CAD build for the part. Positions are in the model's coordinates, mm. Coordinates: 2 decimals unless noted, no trailing zeros. Loops run counter-clockwise (first coordinate to the right, second up) from the corner with the lowest first, then second, coordinate; pieces in that order, holes last. Notation, with made-up numbers: (50.5, 73) -> (95.5, 73) arc R20 ccw to (95.5, 104) -> close; hole circle Ø8 at (-38, -27). An arc over 180 degrees is marked (long way). Write each question's results on one line, items separated by ' | '.
```python
from build123d import *

# Parameters (mm, degrees)
BOSS_EXTRUDE1_DEPTH                             = 6
M3_CLEARANCE_HOLE1_D                            = 3.6
M3_CLEARANCE_HOLE1_DEPTH                        = 6
M3_CLEARANCE_HOLE1_TIP                          = 1.081549114
FILLET1_R                                       = 15
SKETCH4_W                                       = 65
SKETCH4_H                                       = 9
SKETCH4_W_2                                     = 32.5
CUT_EXTRUDE1_DEPTH                              = 2
M4_CLEARANCE_HOLE1_D                            = 4.8
M4_CLEARANCE_HOLE1_DEPTH                        = 6
M4_CLEARANCE_HOLE1_TIP                          = 1.442065486
CHAMFER1_SIZE                                   = 2.4
SKETCH7_W                                       = 65
SKETCH7_H                                       = 78
CUT_EXTRUDE3_DEPTH                              = 132.713704678
FILLET2_R                                       = 15
CSK_FOR_M3_FLAT_HEAD_MACHINE_SCREW1_D           = 3.6
CSK_FOR_M3_FLAT_HEAD_MACHINE_SCREW1_DEPTH       = 20
CSK_FOR_M3_FLAT_HEAD_MACHINE_SCREW1_CSINK_D     = 6.3
CSK_FOR_M3_FLAT_HEAD_MACHINE_SCREW1_CSINK_ANGLE = 90
CSK_FOR_M3_FLAT_HEAD_MACHINE_SCREW1_TIP         = 1.081549114


with BuildPart() as part:
    # Sketch1 → Boss-Extrude1 (new body)
    with BuildSketch(Plane.XY):
        with BuildLine():
            Line((-32.5, 95), (-32.5, -95))
            ThreePointArc((-32.5, -95), (0, -62.5), (32.5, -95))
            Line((32.5, -95), (32.5, 95))
            Line((32.5, 95), (-32.5, 95))
        make_face()
        with BuildLine():
            ThreePointArc((32.5, -95), (0, -62.5), (-32.5, -95))
            Line((-32.5, -95), (-15.5, -95))
            Line((-15.5, -95), (-15.5, -79.5))
            Line((-15.5, -79.5), (15.5, -79.5))
            Line((15.5, -79.5), (15.5, -95))
            Line((15.5, -95), (32.5, -95))
        make_face()
        with BuildLine():
            Line((-15.5, -95), (-32.5, -95))
            ThreePointArc((-32.5, -95), (0, -127.5), (32.5, -95))
            Line((32.5, -95), (15.5, -95))
            Line((15.5, -95), (15.5, -110.5))
            Line((15.5, -110.5), (-15.5, -110.5))
            Line((-15.5, -110.5), (-15.5, -95))
        make_face()
        with BuildLine():
            Line((-14, -95), (-15.5, -95))
            Line((-15.5, -95), (-15.5, -110.5))
            Line((-15.5, -110.5), (15.5, -110.5))
            Line((15.5, -110.5), (15.5, -95))
            Line((15.5, -95), (14, -95))
            ThreePointArc((14, -95), (0, -109), (-14, -95))
        make_face()
        with BuildLine():
            Line((-15.5, -79.5), (-15.5, -95))
            Line((-15.5, -95), (-14, -95))
            ThreePointArc((-14, -95), (0, -81), (14, -95))
            Line((14, -95), (15.5, -95))
            Line((15.5, -95), (15.5, -79.5))
            Line((15.5, -79.5), (-15.5, -79.5))
        make_face()
    extrude(amount=BOSS_EXTRUDE1_DEPTH)

    # M3 Clearance Hole1
    with Locations(Plane(origin=(0, 0, 0), x_dir=(-1, 0, 0), z_dir=(0, 0, -1))):
        with Locations((-15.5, -110.5), (15.5, -110.5), (15.5, -79.5), (-15.5, -79.5)):
            Hole(M3_CLEARANCE_HOLE1_D / 2, depth=M3_CLEARANCE_HOLE1_DEPTH)
            with Locations((0, 0, -(M3_CLEARANCE_HOLE1_DEPTH + M3_CLEARANCE_HOLE1_TIP / 2))):  # 118° drill point
                Cone(0, M3_CLEARANCE_HOLE1_D / 2, M3_CLEARANCE_HOLE1_TIP, mode=Mode.SUBTRACT)

    # Fillet1
    fillet1_edges = [part.edges().sort_by_distance(p)[0] for p in [
        (-32.5, 95, 3),
        (32.5, 95, 3),
    ]]
    fillet(fillet1_edges, radius=FILLET1_R)

    # Sketch4 → Cut-Extrude1 (cut)
    with BuildSketch(Plane.XY.offset(6)):
        with Locations((0, 75.5)):
            Rectangle(SKETCH4_W, SKETCH4_H)
        with Locations((-16.25, 7.5)):
            Rectangle(SKETCH4_W_2, SKETCH4_H)
        with Locations((16.25, 7.5)):
            Rectangle(SKETCH4_W_2, SKETCH4_H)
        with Locations((0, -60.5)):
            Rectangle(SKETCH4_W, SKETCH4_H)
    extrude(amount=-CUT_EXTRUDE1_DEPTH, mode=Mode.SUBTRACT)

    # M4 Clearance Hole1
    with Locations(Plane.XY.offset(4)):
        with Locations((-24.5, -60.5), (-24.5, 75.5), (24.5, 75.5), (0, 75.5), (-24.5, 7.5), (0, 7.5), (24.5, 7.5), (24.5, -60.5), (0, -60.5)):
            Hole(M4_CLEARANCE_HOLE1_D / 2, depth=M4_CLEARANCE_HOLE1_DEPTH)
            with Locations((0, 0, -(M4_CLEARANCE_HOLE1_DEPTH + M4_CLEARANCE_HOLE1_TIP / 2))):  # 118° drill point
                Cone(0, M4_CLEARANCE_HOLE1_D / 2, M4_CLEARANCE_HOLE1_TIP, mode=Mode.SUBTRACT)

    # Chamfer1
    chamfer1_edges = [part.edges().sort_by_distance(p)[0] for p in [
        (-22.1, -60.5, 0),
        (2.4, -60.5, 0),
        (26.9, -60.5, 0),
        (26.9, 7.5, 0),
        (2.4, 7.5, 0),
        (-22.1, 7.5, 0),
        (2.4, 75.5, 0),
        (26.9, 75.5, 0),
        (-22.1, 75.5, 0),
        (13.7, -79.5, 0),
        (-17.3, -79.5, 0),
        (-17.3, -110.5, 0),
        (13.7, -110.5, 0),
    ]]
    chamfer(chamfer1_edges, length=CHAMFER1_SIZE)

    # Sketch7 → Cut-Extrude3 (cut, through all)
    with BuildSketch(Plane.XY.offset(6)):
        with Locations((0, 66)):
            Rectangle(SKETCH7_W, SKETCH7_H)
    extrude(amount=-CUT_EXTRUDE3_DEPTH, mode=Mode.SUBTRACT)

    # Fillet2
    fillet2_edges = [part.edges().sort_by_distance(p)[0] for p in [
        (32.5, 27, 3),
        (-32.5, 27, 3),
    ]]
    fillet(fillet2_edges, radius=FILLET2_R - 0.0001)  # a hair under: the kernel refuses the full size

    # CSK for M3 Flat Head Machine Screw1
    with Locations(Plane(origin=(0, 0, 0), x_dir=(1, 0, 0), z_dir=(0, 0, -1))):
        with Locations((0, 122.3)):
            CounterSinkHole(CSK_FOR_M3_FLAT_HEAD_MACHINE_SCREW1_D / 2, CSK_FOR_M3_FLAT_HEAD_MACHINE_SCREW1_CSINK_D / 2, depth=CSK_FOR_M3_FLAT_HEAD_MACHINE_SCREW1_DEPTH, counter_sink_angle=CSK_FOR_M3_FLAT_HEAD_MACHINE_SCREW1_CSINK_ANGLE)
            with Locations((0, 0, -(CSK_FOR_M3_FLAT_HEAD_MACHINE_SCREW1_DEPTH + CSK_FOR_M3_FLAT_HEAD_MACHINE_SCREW1_TIP / 2))):  # 118° drill point
                Cone(0, CSK_FOR_M3_FLAT_HEAD_MACHINE_SCREW1_D / 2, CSK_FOR_M3_FLAT_HEAD_MACHINE_SCREW1_TIP, mode=Mode.SUBTRACT)


solid = part.part
```
Q1. Drop flat-ended pins along their axis: pin 1 (2.5 mm diameter, centred on x = -3, y = 8, fed in from +Z); pin 2 (0.6 mm diameter, centred on x = -7, z = 4.5, fed in from -Y); pin 3 (22.5 mm diameter, centred on x = 0, y = -95, fed in from +Z); pin 4 (7.5 mm diameter, centred on x = 24.5, y = -60.5, fed in from -Z). Give the stop position or say it passes through.
Results are:
pin 1: z = 4 | pin 2: y = -126.8 | pin 3: through | pin 4: z = 1.05
Q2. Cut at D-D on x = -24. Give the number of separate pieces and of enclosed holes in the cut face, and give its area (3 significant figures).
Results are:
separate pieces: 3 | enclosed holes: 0 | area: 769 mm^2
Q3. Pull direction X, two halves, no side cores. Call faces 1 (the flat face through (-32.5, -41, 3)), 2 (the conical face through (-2.4, 8.26, 2.28)), 3 (the flat face through (0, 27, 3)): +X half, -X half, draft (parallel to the pull), parting line (faces both ways), or undercut.
Results are:
face 1: -X half | face 2: undercut | face 3: draft
Q4. Cut at A-A on y = -60.5. Write the cut outline in (x, z), and give its area (3 significant figures).
Results are:
outline: (-32.5, 0) -> (-29.3, 0) -> (-26.9, 2.4) -> (-26.9, 4) -> (-32.5, 4) -> close; (-22.1, 2.4) -> (-19.7, 0) -> (-4.8, 0) -> (-2.4, 2.4) -> (-2.4, 4) -> (-22.1, 4) -> close; (2.4, 2.4) -> (4.8, 0) -> (19.7, 0) -> (22.1, 2.4) -> (22.1, 4) -> (2.4, 4) -> close; (26.9, 2.4) -> (29.3, 0) -> (32.5, 0) -> (32.5, 4) -> (26.9, 4) -> close | area: 185 mm^2
Q5. Cut at C-C on y = -110.5. Write the cut outline in (x, z).
Results are:
outline: (-28.57, 0) -> (-19.7, 0) -> (-17.3, 2.4) -> (-17.3, 6) -> (-28.57, 6) -> close; (-13.7, 2.4) -> (-11.3, 0) -> (11.3, 0) -> (13.7, 2.4) -> (13.7, 6) -> (-13.7, 6) -> close; (17.3, 2.4) -> (19.7, 0) -> (28.57, 0) -> (28.57, 6) -> (17.3, 6) -> close
Q6. Cut at B-B on x = -15.5. Write the cut outline in (y, z).
Results are:
outline: (-123.57, 0) -> (-114.7, 0) -> (-112.3, 2.4) -> (-112.3, 6) -> (-123.57, 6) -> close; (-108.7, 2.4) -> (-106.3, 0) -> (-83.7, 0) -> (-81.3, 2.4) -> (-81.3, 6) -> (-108.7, 6) -> close; (-77.7, 2.4) -> (-75.3, 0) -> (27, 0) -> (27, 6) -> (12, 6) -> (12, 4) -> (3, 4) -> (3, 6) -> (-56, 6) -> (-56, 4) -> (-65, 4) -> (-65, 6) -> (-77.7, 6) -> close
Q7. Wall check: L1, parallel to X at y = -79.5, z = 4.5; L2, parallel to Y at x = -15.5, z = 3.55; L3, parallel to Y at x = -21.5, z = 4.05. Give the ranges that are in metal, low to high. Write a range as from..to.
Results are:
L1: -32.5..-17.3, -13.7..13.7, 17.3..32.5 | L2: -123.57..-112.3, -108.7..-81.3, -77.7..27 | L3: -119.37..-65, -56..3, 12..26.46
